Build history of the part. All positions in model axes, mm. Face numbers are marked on the shaded views. A direction names the side the tool comes from. Round coordinates to 2 decimals unless told otherwise and drop trailing zeros. Loops run counter-clockwise (first coordinate to the right, second up) from the corner with the lowest first, then second, coordinate; pieces in that order, holes last. Notation, with made-up numbers: M 86,66 L 122,66 A20 cw 122,75 Z; hole C 69,83.5 d3. An arc over 180 degrees is marked long. Use one line per item in the form item = value. Start each with the question number.
```python
from build123d import *

# Parameters (mm, degrees)
EXTRUDE_1_DEPTH             = 0.7
EXTRUDE_2_DEPTH             = 5.5
EXTRUDE_3_DEPTH             = 6.5
SKETCH_4_R                  = 16.7
EXTRUDE_4_DEPTH             = 1.5
EXTRUDE_5_REACH             = 43.838
EXTRUDE_5_START_RADIUS      = 16.7
EXTRUDE_5_END_RADIUS        = 16.7
SKETCH_5_W                  = 30
SKETCH_5_H                  = 12
CUT_EXTRUDE_1_DEPTH         = 5.5
HOLE_WIZARD_2_5_2_5_1_D     = 2.5
HOLE_WIZARD_2_5_2_5_1_DEPTH = 8
HOLE_WIZARD_15_0_15_1_D     = 15
HOLE_WIZARD_15_0_15_1_DEPTH = 14.2
HOLE_WIZARD_3_4_3_4_1_D     = 3.4
HOLE_WIZARD_3_4_3_4_1_DEPTH = 14.2
FILLET_1_R                  = 0.5
FILLET_2_R                  = 2
FILLET_START                = 2
FILLET_3_DEPTH              = 14


with BuildPart() as part:
    # 草图1 → 凸台-拉伸1 (new body)
    with BuildSketch(Plane(origin=(0, 0, 2.3), x_dir=(-1, 0, 0), z_dir=(0, 0, -1))):
        with BuildLine():
            Line((5.499904708, -20.525923809), (4.529333289, -16.90370196))
            ThreePointArc((4.529333289, -16.90370196), (0, -17.5), (-4.529333289, -16.90370196))
            Line((-4.529333289, -16.90370196), (-5.499904708, -20.525923809))
            ThreePointArc((-5.499904708, -20.525923809), (-3.858782139, -20.896705492), (-2.193469574, -21.136489567))
            ThreePointArc((-2.193469574, -21.136489567), (-1.75352934, -20.954121421), (-1.665889964, -20.486013645))
            ThreePointArc((-1.665889964, -20.486013645), (0, -18.2), (1.665889964, -20.486013645))
            ThreePointArc((1.665889964, -20.486013645), (1.75352934, -20.954121421), (2.193469574, -21.136489567))
            ThreePointArc((2.193469574, -21.136489567), (3.858782139, -20.896705492), (5.499904708, -20.525923809))
        make_face()
    extrude(amount=-EXTRUDE_1_DEPTH)

    # 草图2 → 凸台-拉伸2 (add)
    with BuildSketch(Plane.XY.offset(3)):
        with BuildLine():
            Line((-15, -9.013878189), (-15, -7.340980861))
            ThreePointArc((-15, -7.340980861), (0, 16.7), (15, -7.340980861))
            Line((15, -7.340980861), (15, -9.013878189))
            ThreePointArc((15, -9.013878189), (12.1297479, -12.614246544), (8.419780607, -15.341358953))
            ThreePointArc((8.419780607, -15.341358953), (5.738930413, -14.290719986), (4.529333289, -16.90370196))
            Line((4.529333289, -16.90370196), (5.499904708, -20.525923809))
            ThreePointArc((5.499904708, -20.525923809), (3.858782139, -20.896705492), (2.193469574, -21.136489567))
            ThreePointArc((2.193469574, -21.136489567), (1.75352934, -20.954121421), (1.665889964, -20.486013645))
            ThreePointArc((1.665889964, -20.486013645), (0, -18.2), (-1.665889964, -20.486013645))
            ThreePointArc((-1.665889964, -20.486013645), (-1.75352934, -20.954121421), (-2.193469574, -21.136489567))
            ThreePointArc((-2.193469574, -21.136489567), (-3.858782139, -20.896705492), (-5.499904708, -20.525923809))
            Line((-5.499904708, -20.525923809), (-4.529333289, -16.90370196))
            ThreePointArc((-4.529333289, -16.90370196), (-5.738930413, -14.290719986), (-8.419780607, -15.341358953))
            ThreePointArc((-8.419780607, -15.341358953), (-12.1297479, -12.614246544), (-15, -9.013878189))
        make_face()
    extrude(amount=EXTRUDE_2_DEPTH)

    # 草图3 → 凸台-拉伸3 (add)
    with BuildSketch(Plane.XY.offset(8.5)):
        with BuildLine():
            Line((-15, -17.764078923), (-15, -7.340980861))
            ThreePointArc((-15, -7.340980861), (0, 16.7), (15, -7.340980861))
            Line((15, -7.340980861), (15, -17.764078923))
            ThreePointArc((15, -17.764078923), (0, -23.25), (-15, -17.764078923))
        make_face()
    extrude(amount=EXTRUDE_3_DEPTH)

    # 草图4 → 凸台-拉伸4 (add)
    with BuildSketch(Plane.XY.offset(15)):
        with Locations(Location((0, 0, 0), (0, 0, 206.077066929))):
            Circle(SKETCH_4_R)
    extrude(amount=EXTRUDE_4_DEPTH)

    # 凸台-拉伸5: from a cylinder face, 43.838 long prism both ways, kept between that surface and its translate by the depth
    extrude_5_start = Plane(origin=(0, 0, 9), z_dir=(0, 0, -1)) * Cylinder(EXTRUDE_5_START_RADIUS, 122.076, mode=Mode.PRIVATE)
    extrude_5_end = Plane(origin=(0, 10.423098063, 9), z_dir=(0, 0, -1)) * Cylinder(EXTRUDE_5_END_RADIUS, 122.076, mode=Mode.PRIVATE)
    # 草图5 → 凸台-拉伸5 (add, from a surface)
    with BuildSketch(Plane(origin=(0, -4.175, 0), x_dir=(1, 0, 0), z_dir=(0, 1, 0)), mode=Mode.PRIVATE) as extrude_5_sk1:
        with Locations((0, -9)):
            Rectangle(SKETCH_5_W, SKETCH_5_H)
    extrude_5_tool1 = extrude(extrude_5_sk1.sketch, amount=EXTRUDE_5_REACH, both=True, mode=Mode.PRIVATE)
    add(((extrude_5_tool1 - extrude_5_start) & extrude_5_end).solids().sort_by_distance((0, 12.55253, 9))[0])

    # 草图6 → 切除-拉伸1 (cut)
    with BuildSketch(Plane(origin=(0, 0, 3), x_dir=(-1, 0, 0), z_dir=(0, 0, -1))):
        with BuildLine():
            Line((15, 9.013878189), (15, 17.764078923))
            ThreePointArc((15, 17.764078923), (0, 23.25), (-15, 17.764078923))
            Line((-15, 17.764078923), (-15, 9.013878189))
            ThreePointArc((-15, 9.013878189), (0, 17.5), (15, 9.013878189))
        make_face()
    extrude(amount=-CUT_EXTRUDE_1_DEPTH, mode=Mode.SUBTRACT)

    # Ø2.5 (2.5) 直径孔1
    with Locations(Plane(origin=(0, 0, 8.5), x_dir=(-1, 0, 0), z_dir=(0, 0, -1))):
        with Locations((0, -19.95), (11.75, -16.122654868), (-11.75, -16.122654868), (-11.75, 16.122654868), (0, 19.95), (11.75, 16.122654868)):
            Hole(HOLE_WIZARD_2_5_2_5_1_D / 2, depth=HOLE_WIZARD_2_5_2_5_1_DEPTH)

    # Ø15.0 (15) 直径孔1
    with Locations(Plane.XY.offset(16.5)):
        with Locations((0, 0)):
            Hole(HOLE_WIZARD_15_0_15_1_D / 2, depth=HOLE_WIZARD_15_0_15_1_DEPTH)

    # Ø3.4 (3.4) 直径孔1
    with Locations(Plane.XY.offset(16.5)):
        with Locations((11.691342951, -6.75), (11.691342951, 6.75), (0, 13.5), (-11.691342951, 6.75), (-11.691342951, -6.75), (0, -13.5)):
            Hole(HOLE_WIZARD_3_4_3_4_1_D / 2, depth=HOLE_WIZARD_3_4_3_4_1_DEPTH)

    # 圆角1
    fillet_1_edges = [part.edges().sort_by_distance(p)[0] for p in [
        (5.499904708, -20.525923809, 5.4),
        (4.529333289, -16.90370196, 2.65),
        (-4.529333289, -16.90370196, 2.65),
        (-5.499904708, -20.525923809, 5.4),
        (-8.419780607, -15.341358953, 5.75),
        (8.419780607, -15.341358953, 5.75),
    ]]
    fillet(fillet_1_edges, radius=FILLET_1_R)

    # 圆角2
    # the kernel refuses this fillet: 2 mm, written as the material it adds along each edge
    with BuildSketch(Plane(origin=(15, -7.340980861, 3), x_dir=(0, -1, 0), z_dir=(0, 0, 1)), Plane(origin=(-15, -7.340980861, 15), x_dir=(0, -1, 0), z_dir=(0, 0, -1))) as fillet_2_piece_1:
        with BuildLine():
            CenterArc((0.449397821, 2), FILLET_2_R, 245.380022671, 24.619977329)
            ThreePointArc((-0.38379776, 0.181818182), (-0.191320895, 0.092129153), (0, 0))
            Line((0, 0), (0.449397821, 0))
        make_face()
    extrude(amount=12)
    with BuildSketch(Plane(origin=(-15, 7.340980861, 15), x_dir=(-0.4281233512586551, -0.9037203085618128, 0), z_dir=(0, 0, -1))) as fillet_2_piece_2:
        with BuildLine():
            CenterArc((0.450116765, 1.999838318), FILLET_2_R, 244.651477871, 24.619977329)
            Line((-0.406129937, 0.192397701), (0, 0))
            ThreePointArc((0, 0), (0.21234322, 0.001350044), (0.42468644, 0))
        make_face()
    extrude(amount=12)
    with BuildSketch(Plane(origin=(15, 7.340980861, 15), x_dir=(0.4281233512586662, -0.9037203085618076, 0), z_dir=(0, 0, -1))) as fillet_2_piece_3:
        with BuildLine():
            CenterArc((0.450116765, -1.999838318), FILLET_2_R, 90.7285448, 24.619977329)
            Line((-0.406129937, -0.192397701), (0, 0))
            ThreePointArc((0, 0), (0.21234322, -0.001350044), (0.42468644, 0))
        make_face()
    extrude(amount=12)
    # the kernel refuses this fillet: 2 mm, written as the material it takes off along each edge
    with BuildSketch(Plane(origin=(-15, 9.013878189, 1.478131702), x_dir=(0, -1, 0), z_dir=(0, 0, 1))) as fillet_2_2_piece_1:
        with BuildLine():
            CenterArc((0.572906681, 2), FILLET_2_R, 237.004114526, 32.995885474)
            ThreePointArc((-0.516250933, 0.322580645), (-0.259528216, 0.159045393), (0, 0))
            Line((0, 0), (0.572906681, 0))
        make_face()
    extrude(amount=7.021868298, mode=Mode.SUBTRACT)
    with BuildSketch(Plane(origin=(15, 9.013878189, 1.478131702), x_dir=(0, -1, 0), z_dir=(0, 0, 1)), Plane(origin=(-15, -9.013878189, 1.478131702), x_dir=(0, 1, 0), z_dir=(0, 0, 1))) as fillet_2_2_piece_2:
        with BuildLine():
            CenterArc((0.572906681, -2), FILLET_2_R, 90, 32.995885474)
            ThreePointArc((-0.516250933, -0.322580645), (-0.259528216, -0.159045393), (0, 0))
            Line((0, 0), (0.572906681, 0))
        make_face()
    extrude(amount=7.021868298, mode=Mode.SUBTRACT)
    with BuildSketch(Plane(origin=(15, -9.013878189, 1.478131702), x_dir=(-0.5299089374298662, -0.8480545489719102, 0), z_dir=(0, 0, 1))) as fillet_2_2_piece_3:
        with BuildLine():
            CenterArc((0.573961758, -1.999697468), FILLET_2_R, 89.00341683, 32.995885474)
            Line((-0.485856117, -0.30358837), (0, 0))
            ThreePointArc((0, 0), (0.30437366, 0.002647152), (0.608747319, 0))
        make_face()
    extrude(amount=7.021868298, mode=Mode.SUBTRACT)

    # 圆角3: read off the stored shape, not the designer's step
    # 圆角3 outline → 圆角3 (cut)
    with BuildSketch(Plane.XY.offset(FILLET_START)):
        with BuildLine():
            ThreePointArc((15, 17.764078923), (14.799825954, 18.159709189), (14.589219331, 18.549885824))
            ThreePointArc((14.589219331, 18.549885824), (14.895628938, 17.785343438), (15, 16.968325331))
            Line((15, 16.968325331), (15, 17.764078923))
        make_face()
        with BuildLine():
            ThreePointArc((-14.589219331, 18.549885824), (-14.799825954, 18.159709189), (-15, 17.764078923))
            Line((-15, 17.764078923), (-15, 16.968325331))
            ThreePointArc((-15, 16.968325331), (-14.895628938, 17.785343438), (-14.589219331, 18.549885824))
        make_face()
        with BuildLine():
            Line((15, -17.764078923), (15, -16.18448331))
            ThreePointArc((15, -16.18448331), (14.645511073, -17.660462857), (13.659375, -18.814461847))
            ThreePointArc((13.659375, -18.814461847), (14.339308558, -18.301549936), (15, -17.764078923))
        make_face()
        with BuildLine():
            ThreePointArc((-15, -17.764078923), (-14.339308558, -18.301549936), (-13.659375, -18.814461847))
            ThreePointArc((-13.659375, -18.814461847), (-14.645511073, -17.660462857), (-15, -16.18448331))
            Line((-15, -16.18448331), (-15, -17.764078923))
        make_face()
    extrude(amount=FILLET_3_DEPTH, mode=Mode.SUBTRACT)


solid = part.part
```
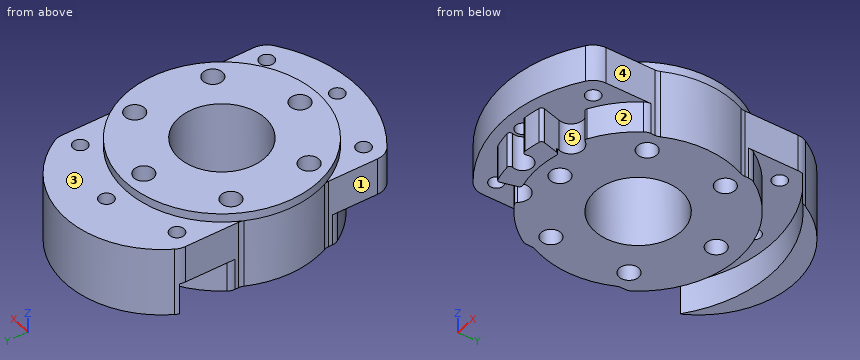
Q1. Tool access for the marked faces 1, 2, 3, 4 and 5: list every direction of +Z, -Z, +X, -X, +Y, -Y with a clear straight run to the whole face (end or side of a thin tool).
Q2. Drop flat-ended pins along their axis: P1, Ø2, axis at y = 11.5, z = 13.5, coming from the -X side; P2, Ø3, axis at x = -11.75, y = -16.12, coming from the -Z side; P3, Ø6, axis at x = 2.5, z = 10.5, coming from the -Y side; P4, Ø7.5, axis at x = 5.5, y = 23.5, coming from the -Z side. Give the stop position or say it passes through.
Q3. Wall check: probe 1 along X at (y, z) = (16, 9); probe 2 along Y at (x, z) = (0, 10.25); probe 3 along Y at (x, z) = (1, 12.5). Give the ranges that are in metal, low to high.
Q4. Saw through at B-B (x = -11.75). Give the number of separate pieces and of enclosed holes in the cut face, and give its area (3 significant figures).
Q5. Saw through at A-A (y = 0). Give the cut face in (x, z), and give its area (3 significant figures).
Filled in:
q1.face_1 = +Z, -Z, -X, -Y
q1.face_2 = -Z, +X, -Y
q1.face_3 = +Z, +Y
q1.face_4 = +Z, -Z, +X, -Y
q1.face_5 = -Z
q2.P1 = -15
q2.P2 = 8.5
q2.P3 = -23.25
q2.P4 = 3
q3.probe_1 = -15 to -12.99, -10.51 to 10.51, 12.99 to 15
q3.probe_2 = -23.25 to -21.2, -18.7 to -15.2, -11.8 to -7.5, 7.5 to 11.8, 15.2 to 18.7, 21.2 to 27.12
q3.probe_3 = -23.23 to -20.7, -19.2 to -14.87, -12.13 to -7.43, 7.43 to 12.13, 14.87 to 19.2, 20.7 to 27.09
q4.separate_pieces = 5
q4.enclosed_holes = 0
q4.area = 342 mm²
q5.outline = M -16.7,3 L -7.5,3 L -7.5,16.5 L -16.7,16.5 Z; M 7.5,3 L 16.7,3 L 16.7,16.5 L 7.5,16.5 Z
q5.area = 248 mm²
